from build123d import *

# Parameters (mm, degrees)
BASE_SKETCH_W                    = 15
BASE_SKETCH_H                    = 15
BASE_SKETCH_EXTRUDE_DEPTH        = 25
CENTER_NUB_CUTOUT_SKETCH_W       = 3.5
CENTER_NUB_CUTOUT_SKETCH_H       = 15
HINGE_NUB_EXTRUDED_CUT_DEPTH     = 12
HINGE_CUTOUT_SKETCH_W            = 10
HINGE_CUTOUT_SKETCH_H            = 15
HINGE_CUTOUT_EXTRUDED_CUT_DEPTH  = 12
HINGE_HOLE_SKETCH_R              = 1
HINGE_HOLE_EXTRUDED_CUT_DEPTH    = 31.103986447
CORNER_FILLETS_R                 = 5
STYLE_FILLETS_R                  = 1
ROUTING_HOLES_SKETCH_W           = 5
ROUTING_HOLES_SKETCH_H           = 2
ROUTING_HOLES_EXTRUDED_CUT_DEPTH = 28.156951228
SKETCH1_W                        = 10
SKETCH1_H                        = 2
BACKING_EXTRUDE_DEPTH            = 6.75
EXTRA_ROUTING_CUT_SKETCH_W       = 5
EXTRA_ROUTING_CUT_SKETCH_H       = 10
EXTRA_ROUTING_EXTRUDED_CUT_DEPTH = 4
ROUTING_FILLETS_R                = 1


with BuildPart() as part:
    # Base Sketch → Base Sketch Extrude (new body)
    with BuildSketch(Plane.XY):
        Rectangle(BASE_SKETCH_W, BASE_SKETCH_H)
    extrude(amount=BASE_SKETCH_EXTRUDE_DEPTH)

    # Center Nub Cutout Sketch → Hinge Nub Extruded Cut (cut)
    with BuildSketch(Plane.XY):
        with Locations((5.75, 0)):
            Rectangle(CENTER_NUB_CUTOUT_SKETCH_W, CENTER_NUB_CUTOUT_SKETCH_H)
        with Locations((-5.75, 0)):
            Rectangle(CENTER_NUB_CUTOUT_SKETCH_W, CENTER_NUB_CUTOUT_SKETCH_H)
    extrude(amount=HINGE_NUB_EXTRUDED_CUT_DEPTH, mode=Mode.SUBTRACT)

    # Hinge Cutout Sketch → Hinge Cutout Extruded Cut (cut)
    with BuildSketch(Plane.XY.offset(25)):
        Rectangle(HINGE_CUTOUT_SKETCH_W, HINGE_CUTOUT_SKETCH_H)
    extrude(amount=-HINGE_CUTOUT_EXTRUDED_CUT_DEPTH, mode=Mode.SUBTRACT)

    # Hinge Hole Sketch → Hinge Hole Extruded Cut (cut, through all)
    with BuildSketch(Plane(origin=(7.5, 0, 0), x_dir=(0, 0, -1), z_dir=(1, 0, 0))):
        with Locations(Location((-5, 0, 0), (0, 0, 90))):
            Circle(HINGE_HOLE_SKETCH_R)
        with Locations(Location((-22, 0, 0), (0, 0, 90))):
            Circle(HINGE_HOLE_SKETCH_R)
    extrude(amount=-HINGE_HOLE_EXTRUDED_CUT_DEPTH, mode=Mode.SUBTRACT)

    # Corner Fillets
    corner_fillets_edges = [part.edges().sort_by_distance(p)[0] for p in [
        (0, -7.5, 0),
        (0, 7.5, 0),
        (-6.25, -7.5, 25),
        (-6.25, 7.5, 25),
        (6.25, -7.5, 25),
        (6.25, 7.5, 25),
    ]]
    fillet(corner_fillets_edges, radius=CORNER_FILLETS_R)

    # Style Fillets
    style_fillets_edges = [part.edges().sort_by_distance(p)[0] for p in [
        (4, 7.5, 8.5),
        (4, -7.5, 8.5),
        (7.5, 0, 12),
        (5.75, 7.5, 12),
        (4, 0, 12),
        (5.75, -7.5, 12),
        (-4, -7.5, 8.5),
        (-4, 7.5, 8.5),
        (-7.5, 0, 12),
        (-5.75, -7.5, 12),
        (-4, 0, 12),
        (-5.75, 7.5, 12),
        (-7.5, 0, 25),
        (-7.5, -7.5, 16),
        (7.5, -7.5, 16),
        (-7.5, 7.5, 16),
        (-7.5, 6.035533906, 23.535533906),
        (-7.5, -6.035533906, 23.535533906),
        (7.5, 7.5, 16),
        (7.5, 0, 25),
        (7.5, 6.035533906, 23.535533906),
        (7.5, -6.035533906, 23.535533906),
        (4, 0, 0),
        (4, 6.035533906, 1.464466094),
        (4, -6.035533906, 1.464466094),
        (-4, 0, 0),
        (-4, 6.035533906, 1.464466094),
        (-4, -6.035533906, 1.464466094),
    ]]
    fillet(style_fillets_edges, radius=STYLE_FILLETS_R)

    # Routing Holes Sketch → Routing Holes Extruded Cut (cut, through all)
    with BuildSketch(Plane.XY):
        with Locations((0, 4.5)):
            Rectangle(ROUTING_HOLES_SKETCH_W, ROUTING_HOLES_SKETCH_H)
        with Locations((0, -4.5)):
            Rectangle(ROUTING_HOLES_SKETCH_W, ROUTING_HOLES_SKETCH_H)
    extrude(amount=ROUTING_HOLES_EXTRUDED_CUT_DEPTH, mode=Mode.SUBTRACT)

    # Sketch1 → Backing Extrude (add)
    with BuildSketch(Plane.XY.offset(13)):
        with Locations((0, -6.5)):
            Rectangle(SKETCH1_W, SKETCH1_H)
    extrude(amount=BACKING_EXTRUDE_DEPTH)

    # Extra Routing Cut Sketch → Extra Routing Extruded Cut (cut)
    with BuildSketch(Plane(origin=(0, 7.5, 0), x_dir=(1, 0, 0), z_dir=(0, 1, 0))):
        with Locations((0, -6)):
            Rectangle(EXTRA_ROUTING_CUT_SKETCH_W, EXTRA_ROUTING_CUT_SKETCH_H)
    extrude(amount=-EXTRA_ROUTING_EXTRUDED_CUT_DEPTH, mode=Mode.SUBTRACT)

    # Routing Fillets
    routing_fillets_edges = [part.edges().sort_by_distance(p)[0] for p in [
        (0, -3.5, 0.101020514),
        (2.5, -4.5, 13),
        (0, -3.5, 13),
        (-2.5, -4.5, 13),
        (2.5, 4.5, 13),
        (0, 3.5, 13),
        (-2.5, 4.5, 13),
        (0, 5.5, 13),
        (0, 5.5, 11),
    ]]
    fillet(routing_fillets_edges, radius=ROUTING_FILLETS_R - 0.0001)  # a hair under: the kernel refuses the full size


solid = part.part
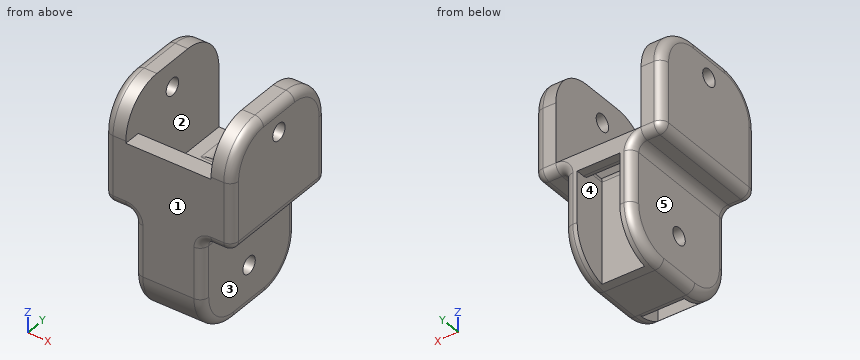
The listing builds one solid part. Answer for the finished solid, in the listing's coordinates (mm). Face numbers are marked on the shaded views. A direction names the side the tool comes from. Round coordinates to 2 decimals unless told otherwise and drop trailing zeros. Write each loop counter-clockwise with the first axis right and the second up, starting at its lowest first coordinate (ties: lowest second). Pieces come first, ordered by that corner, then holes. Notation, with made-up numbers: M 68.25,47.25 L 82.25,47.25 A13 cw 82.25,55.25 Z; hole C 61.5,-40 d11. An arc over 180 degrees is marked long. Write each question's results on one line, items separated by ' | '. Start each with the question number.
(1) The part is cut by section A-A, the plane y = 0. Give the number of separate pieces and of enclosed holes in the cut face, and give its area (3 significant figures).
(2) For the marked faces 1 and 2, determine the directions among +Z, -Z, +X, -X, +Y, -Y from which every point of the face is accessible in a straight line to the end or side of a thin tool.
(3) Determine the mould class of the marked faces 3, 4 and 5 for opening direction X: +X half, -X half, draft (parallel to the pull), parting line (faces both ways), or undercut.
(4) The part is cut by section C-C, the plane z = 17.25. Write down the section's boundary in (x, y), and give its area (3 significant figures).
(5) Each of these flat-tipped pins is pushed along its axis until it touches: P1, Ø2, axis at y = 4.5, z = 8.5, coming from the +X side; P2, Ø6, axis at x = -0.5, z = 19.5, coming from the +Y side; P3, Ø5, axis at y = -1.5, z = 6, coming from the -X side. Where does it stop, or does it pass through?
(6) Find the intervals of material crossed by line 1 (X direction, y = 1.5, z = 18.25); line 2 (Z direction, x = -6.4, y = 0); line 3 (X direction, y = 5.25, z = 5.5), in increasing order.
(7) The part is cut by section D-D, the plane y = 1.75. Write down the section's boundary in (x, z).
Worked answers:
1) separate pieces: 4 | enclosed holes: 0 | area: 144 mm²
2) face 1: +Z, -Z, +X, -X, -Y | face 2: +Z, +Y
3) face 3: +X half | face 4: undercut | face 5: -X half
4) outline: M -7.5,-6.5 A1 ccw -6.5,-7.5 L 6.5,-7.5 A1 ccw 7.5,-6.5 L 7.5,6.5 A1 ccw 6.5,7.5 L 5,7.5 L 5,-5.5 L -5,-5.5 L -5,7.5 L -6.5,7.5 A1 ccw -7.5,6.5 Z | area: 94.1 mm²
5) P1: stops at x = 4 | P2: stops at y = -5.5 | P3: stops at x = -4
6) line 1: x = -7.5 to -5, 5 to 7.5 | line 2: z = 12 to 21, 23 to 25 | line 3: x = -4 to -2.5, 2.5 to 4
7) outline: M -7.5,13 A1 ccw -6.5,12 L -5,12 A1 cw -4,11 L -4,1 A1 ccw -3,0 L 3,0 A1 ccw 4,1 L 4,11 A1 cw 5,12 L 6.5,12 A1 ccw 7.5,13 L 7.5,24 A1 ccw 6.5,25 L 5,25 L 5,13 L -5,13 L -5,25 L -6.5,25 A1 ccw -7.5,24 Z
